The drawing under review shows one solid part. Ordinate dimensions are in mm from its lowest x, y, z. A direction names the side the tool comes from. Coordinates: 2 decimals unless noted, no trailing zeros. Order: outer loops, then holes, each group sorted by start corner. A loop starts at its lowest first (then second) coordinate and runs counter-clockwise, first axis right, second up.
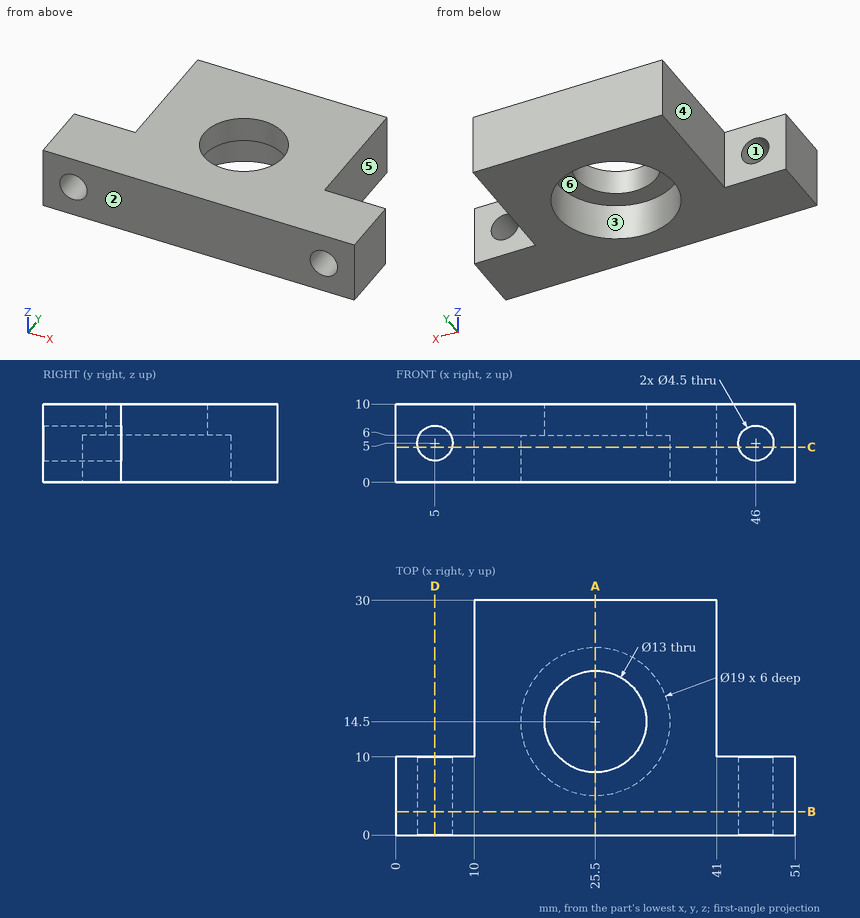
1. Machinability: for the marked faces 4, 5 and 6, which of the approach directions +Z, -Z, +X, -X, +Y, -Y give a long, thin tool a straight path to every point of the face, cutting with its end or side? Answer none if there is none.
Answer below:
face 4: +Z, -Z, -X, +Y
face 5: +Z, -Z, +X, +Y
face 6: -Z
2. Take a section at C-C, the plane z = 4.5. Give the boundary of the cut face in (x, y).
Answer below:
outline: (0, 0) - (2.81, 0) - (2.81, 10) - (0, 10) - close; (7.19, 0) - (43.81, 0) - (43.81, 10) - (41, 10) - (41, 30) - (10, 30) - (10, 10) - (7.19, 10) - close; (48.19, 0) - (51, 0) - (51, 10) - (48.19, 10) - close; hole circle Ø19 at (25.5, 14.5)
3. The part is to be moulded in two halves that separate along Y. For the marked faces 1, 2 and 3, say which applies: +Y half, -Y half, draft (parallel to the pull), parting line (faces both ways), or undercut.
Answer below:
face 1: draft
face 2: -Y half
face 3: undercut
4. Take a section at B-B, the plane y = 3. Give the boundary of the cut face in (x, z).
Answer below:
outline: (0, 0) - (51, 0) - (51, 10) - (0, 10) - close; hole circle Ø4.5 at (5, 5); hole circle Ø4.5 at (46, 5)
5. Take a section at D-D, the plane x = 5. Give the boundary of the cut face in (y, z).
Answer below:
outline: (0, 0) - (10, 0) - (10, 2.75) - (0, 2.75) - close; (0, 7.25) - (10, 7.25) - (10, 10) - (0, 10) - close
6. Clearance check with flat-ended pins moving along their axes: pin 1 Ø6 at (x, z) = (46, 5) entering from +Y; pin 2 Ø9.5 at (x, y) = (25.5, 14) entering from -Z; pin 3 Ø3 at (y, z) = (17.5, 7.5) entering from +X. State where each tip first meets the part, or that it passes through.
Answer below:
pin 1: stops at y = 10
pin 2: passes through
pin 3: stops at x = 41
7. Take a section at A-A, the plane x = 25.5. Give the boundary of the cut face in (y, z), plus the area to 3 significant figures.
Answer below:
outline: (0, 0) - (5, 0) - (5, 6) - (8, 6) - (8, 10) - (0, 10) - close; (21, 6) - (24, 6) - (24, 0) - (30, 0) - (30, 10) - (21, 10) - close
area: 134 mm2
8. To check wall thickness, follow L1, parallel to Z at x = 46, y = 5; L2, parallel to Y at x = 25.5, z = 1.45; L3, parallel to Z at x = 30.5, y = 6.5. State the ranges of each line that lie inside material, in increasing order.
Answer below:
L1: z = 0 to 2.75, 7.25 to 10
L2: y = 0 to 5, 24 to 30
L3: z = 6 to 10
